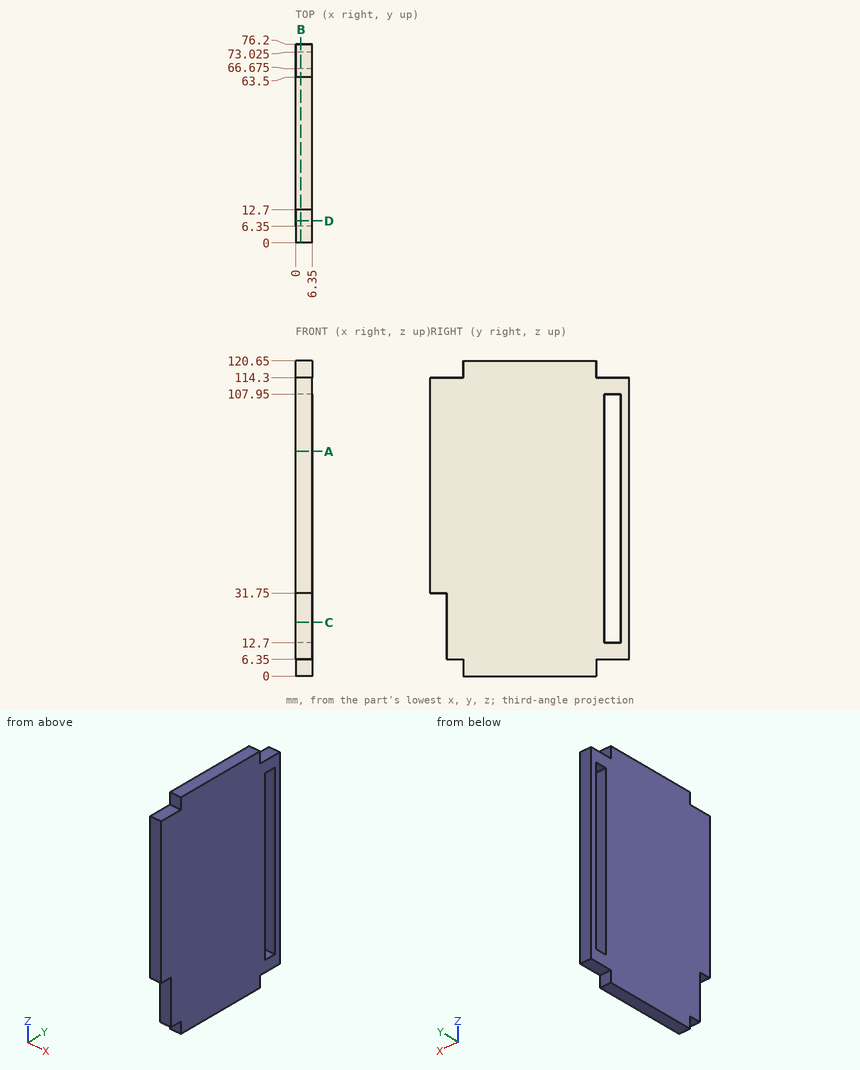
Geometry: see drawing. Coordinates: mm, zero at the bounding-box minimum. Coordinates: 2 decimals unless noted, no trailing zeros. Write each loop counter-clockwise with the first axis right and the second up, starting at its lowest first coordinate (ties: lowest second). Pieces come first, ordered by that corner, then holes. Notation, with made-up numbers: (70, -33) - (100, -33) arc R28 cw to (100, -4) - close; hole circle Ø11 at (30, -26). An arc over 180 degrees is marked (long way). Put each result on its own line as item: value. Start each with the question number.
1) Cut plane A-A (z = 86). Return the cut outline in (x, y) (3 decimals), plus the area to 3 significant figures.
2) Cut plane D-D (y = 8.5). Return the cut outline in (x, z), plus the area to 3 significant figures.
3) Contact query for flat-ended pins moving along their axis: pin 1 (1.9 mm diameter, centred on x = 2.5, y = 72.5, fed in from -Z); pin 2 (3 mm diameter, centred on x = 3, y = 3, fed in from -Z); pin 3 (3 mm diameter, centred on x = 4, z = 3, fed in from -Y). Output: stop coordinate, or through.
4) Ray query, L1, parallel to Y at x = 6, z = 95.5 (3 decimals); L2, parallel to Z at x = 2.75, y = 68; L3, parallel to Z at x = 2.75, y = 10.5. Return the intervals inside material, ascending.
5) Cut plane C-C (z = 20.5). Return the cut outline in (x, y) (3 decimals), plus the area to 3 significant figures.
6) Cut plane B-B (x = 2). Return the cut outline in (y, z) (3 decimals), plus the area to 3 significant figures.
Resolved:
1. outline: (0, 0) - (6.35, 0) - (6.35, 66.675) - (0, 66.675) - close; (0, 73.025) - (6.35, 73.025) - (6.35, 76.2) - (0, 76.2) - close
1. area: 444 mm2
2. outline: (0, 6.35) - (6.35, 6.35) - (6.35, 114.3) - (0, 114.3) - close
2. area: 685 mm2
3. pin 1: stops at z = 6.35
3. pin 2: stops at z = 31.75
3. pin 3: stops at y = 12.7
4. L1: y = 0 to 66.675, 73.025 to 76.2
4. L2: z = 6.35 to 12.7, 107.95 to 114.3
4. L3: z = 6.35 to 114.3
5. outline: (0, 6.35) - (6.35, 6.35) - (6.35, 66.675) - (0, 66.675) - close; (0, 73.025) - (6.35, 73.025) - (6.35, 76.2) - (0, 76.2) - close
5. area: 403 mm2
6. outline: (0, 31.75) - (6.35, 31.75) - (6.35, 6.35) - (12.7, 6.35) - (12.7, 0) - (63.5, 0) - (63.5, 6.35) - (76.2, 6.35) - (76.2, 114.3) - (63.5, 114.3) - (63.5, 120.65) - (12.7, 120.65) - (12.7, 114.3) - (0, 114.3) - close; hole (66.675, 12.7) - (73.025, 12.7) - (73.025, 107.95) - (66.675, 107.95) - close
6. area: 8,100 mm2
